Geometry: final body of the model. Coordinates: model frame, mm. A direction names the side the tool comes from. Give positions to 0.01 mm unless a question says otherwise; leave off trailing zeros. Loops run counter-clockwise (first coordinate to the right, second up) from the corner with the lowest first, then second, coordinate; pieces in that order, holes last. Notation, with made-up numbers: (78, 3.5) - (109, 3.5) arc R12 ccw to (109, 10.5) - close; hole circle Ø6 at (4.5, -6.75). An arc over 180 degrees is marked (long way). Use one line per item in the form item = value.
```python
from build123d import *

# Parameters (mm, degrees)
F0_R      = 8.5
F1_DEPTH  = 4
F3_R      = 5
F4_DEPTH  = 100
F5_W      = 4
F5_H      = 5
F9_R      = 1
F10_DEPTH = 5
F11_R     = 1.5
F12_DEPTH = 128.4


with BuildPart() as f1:
    # F0 (on Top) → F1 (new body)
    with BuildSketch(Plane.XY):
        Circle(F0_R)
    extrude(amount=F1_DEPTH)

    # F3 (on Top) → F4 (join)
    with BuildSketch(Plane.XY):
        Circle(F3_R)
    extrude(amount=F4_DEPTH)

    # F5 (on Right) → F6 (revolve)
    with BuildSketch(Plane.YZ):
        with Locations((2, 102.5)):
            Rectangle(F5_W, F5_H)
    revolve(axis=Axis((0, 0, 102.5), (0, 0, -1)))

    # F9 (on face) → F10 (join)
    with BuildSketch(Plane.YZ.offset(8.440972)):
        with Locations((0, 2)):
            Circle(F9_R)
    extrude(amount=F10_DEPTH)

    # F11 (on face) → F12 (cut)
    with BuildSketch(Plane.XY.offset(105)):
        Circle(F11_R)
    extrude(amount=-F12_DEPTH, mode=Mode.SUBTRACT)


solid = f1.part
```
(1) Cut plane D-D (y = 7.25). Return the cut outline in (x, z), plus the area to 3 significant figures.
Solution:
outline = (-4.44, 0) - (4.44, 0) - (4.44, 4) - (-4.44, 4) - close
area = 35.5 mm2
(2) Pin query (flat end, axial travel): P1, Ø3, axis at x = 3, z = 42, coming from the -Y side; P2, Ø2, axis at y = 4, z = 62, coming from the +X side; P3, Ø4, axis at x = 7.5, y = 5.5, coming from the -Z side; P4, Ø5, axis at y = 4.5, z = 29.5, coming from the +X side. Return the tip coordinate at first contact, or that it passes through.
Solution:
P1 = -4.77
P2 = 4
P3 = 0
P4 = 4.58
(3) Cut plane A-A (x = 0). Return the cut outline in (y, z), plus the area to 3 significant figures.
Solution:
outline = (-8.5, 0) - (-1.5, 0) - (-1.5, 105) - (-4, 105) - (-4, 100) - (-5, 100) - (-5, 4) - (-8.5, 4) - close; (1.5, 0) - (8.5, 0) - (8.5, 4) - (5, 4) - (5, 100) - (4, 100) - (4, 105) - (1.5, 105) - close
area = 753 mm2
(4) Access query for faces 1 (the face through (2, 0, 0)), 2 (the face through (11, 0, 1)), 3 (the face through (-3.905, -0.867, 102.535)). Directions: +Z, -Z, +X, -X, +Y, -Y. A direction counts if a zero-diameter tool reaches every point of the face in a straight line with its end or side. Return the directions, or none.
Solution:
face_1 = -Z, +X, -X, +Y, -Y
face_2 = +X
face_3 = +Z
(5) Material intervals for L1, parallel to Y at x = 0, z = 33.5; L2, parallel to Z at x = -6.25, y = 2.5; L3, parallel to Z at x = -4.75, y = -0.5, sorted ascending. Write a range as from..to.
Solution:
L1 = -5..-1.5, 1.5..5
L2 = 0..4
L3 = 0..100
(6) Pull-direction query (X, two-part tool) for faces 4 (the face through (13.441, 0, 2)), 5 (the face through (-1.5, 0.07, 53.24)), 6 (the face through (4, -4, 4)), 7 (the face through (4.57, 7.167, 1.972)); classes: released by +X, released by -X, zero draft, split by the parting line, or undercut.
Solution:
face_4 = released by +X
face_5 = undercut
face_6 = zero draft
face_7 = split by the parting line
(7) Cut plane B-B (y = 0). Return the cut outline in (x, z).
Solution:
outline = (-8.5, 0) - (-1.5, 0) - (-1.5, 105) - (-4, 105) - (-4, 100) - (-5, 100) - (-5, 4) - (-8.5, 4) - close; (1.5, 0) - (8.5, 0) - (8.5, 1) - (13.44, 1) - (13.44, 3) - (8.5, 3) - (8.5, 4) - (5, 4) - (5, 100) - (4, 100) - (4, 105) - (1.5, 105) - close
(8) Cut plane C-C (z = 42). Return the cut outline in (x, y).
Solution:
outline = circle Ø10 at (0, 0); hole circle Ø3 at (0, 0)
